from build123d import *

# Parameters (mm, degrees)
SKETCH1_R           = 5
BOSS_EXTRUDE1_DEPTH = 40
SKETCH1_3_R         = 7.5
SKETCH1_3_R_2       = 5
BOSS_EXTRUDE2_DEPTH = 3
SKETCH2_R           = 7.5
BOSS_EXTRUDE3_DEPTH = 7


with BuildPart() as part:
    # Sketch1 → Boss-Extrude1 (new body)
    with BuildSketch(Plane(origin=(0, 0, 0), x_dir=(1, 0, 0), z_dir=(0, 1, 0))):
        with Locations(Location((0, 0, 0), (0, 0, 270))):
            Circle(SKETCH1_R)
    extrude(amount=BOSS_EXTRUDE1_DEPTH)

    # Sketch1_3 → Boss-Extrude2 (add)
    with BuildSketch(Plane(origin=(0, 0, 0), x_dir=(1, 0, 0), z_dir=(0, 1, 0))):
        with Locations(Location((0, 0, 0), (0, 0, 270))):
            Circle(SKETCH1_3_R)
        Polygon((2.886751346, -5), (5.773502692, 0), (2.886751346, 5), (-2.886751346, 5), (-5.773502692, 0), (-2.886751346, -5), align=None, mode=Mode.SUBTRACT)
        with BuildLine():
            ThreePointArc((-4.330127013, 2.500000011), (-2.499999995, 4.330127022), (0, 5))
            Line((0, 5), (-2.886751346, 5))
            Line((-2.886751346, 5), (-4.330127013, 2.500000011))
        make_face()
        with BuildLine():
            ThreePointArc((0, 5), (2.500000021, 4.330127007), (4.330127043, 2.499999958))
            Line((4.330127043, 2.499999958), (2.886751346, 5))
            Line((2.886751346, 5), (0, 5))
        make_face()
        with BuildLine():
            Line((4.330126994, -2.500000043), (5.773502692, 0))
            Line((5.773502692, 0), (4.330127043, 2.499999958))
            ThreePointArc((4.330127043, 2.499999958), (4.829629138, 1.294095202), (5, 0))
            ThreePointArc((5, 0), (4.829629125, -1.294095249), (4.330126994, -2.500000043))
        make_face()
        with BuildLine():
            Line((2.886751346, -5), (4.330126994, -2.500000043))
            ThreePointArc((4.330126994, -2.500000043), (2.499999979, -4.330127031), (0, -5))
            Line((0, -5), (2.886751346, -5))
        make_face()
        with BuildLine():
            Line((-2.886751346, -5), (0, -5))
            ThreePointArc((0, -5), (-2.499999995, -4.330127022), (-4.330127013, -2.500000011))
            Line((-4.330127013, -2.500000011), (-2.886751346, -5))
        make_face()
        with BuildLine():
            ThreePointArc((-4.330127013, -2.500000011), (-5, 0), (-4.330127013, 2.500000011))
            Line((-4.330127013, 2.500000011), (-5.773502692, 0))
            Line((-5.773502692, 0), (-4.330127013, -2.500000011))
        make_face()
        with Locations(Location((0, 0, 0), (0, 0, 270))):
            Circle(SKETCH1_3_R_2)
    extrude(amount=-BOSS_EXTRUDE2_DEPTH)

    # Sketch2 → Boss-Extrude3 (add)
    with BuildSketch(Plane.XZ.offset(3)):
        with Locations(Location((0, 0, 0), (0, 0, 90))):
            Circle(SKETCH2_R)
        Polygon((5.773502692, 0), (2.886751346, 5), (-2.886751346, 5), (-5.773502692, 0), (-2.886751346, -5), (2.886751346, -5), align=None, mode=Mode.SUBTRACT)
    extrude(amount=BOSS_EXTRUDE3_DEPTH)


solid = part.part
Verification items for the finished model (mm, model axes). A direction names the side the tool comes from. Coordinates: 2 decimals unless noted, no trailing zeros. Order: outer loops, then holes, each group sorted by start corner. A loop starts at its lowest first (then second) coordinate and runs counter-clockwise, first axis right, second up. Notation, with made-up numbers: (-11, 18) -> (4, 18) arc R34 cw to (4, 54) -> close; hole circle Ø3 at (83.5, 3). An arc over 180 degrees is marked (long way). Put each result on its own line as item: value. Start each with the question number.
1. Cross-section at B-B, the plane y = 9. Record the boundary of the cut face in (x, z).
2. Access from +Z, -Z, +X, -X, +Y, -Y to the whole of each face (thin tool, end or side, straight path). Record for faces 5 (the cylindrical face through (-0.33, -4.93, -7.493)), 6 (the flat face through (-5, 0, 2)), 7 (the flat face through (-4.35, -6.451, -2.465)).
3. Material ranges on L1, parallel to Y at x = -1.25, z = -2.75; L2, parallel to Y at x = 4, z = -5; L3, parallel to Z at x = -0.75, y = -6.5, recorded low to high. Write a range as [from, to].
4. Mould release check, pull along Z, two halves, no side actions. Record for faces 1 (the flat face through (0, -6, 5)), 2 (the cylindrical face through (-4.88, 19.72, -1.08)), 3 (the flat face through (4.31, -6.451, -2.535)), 4 (the flat face through (5, -10, -2)): released by +Z, released by -Z, zero draft, split by the parting line, or undercut.
5. Go/stop test with flat-tipped pins: pin 1 Ø5 at (x, y) = (-3, 26) entering from +Z; pin 2 Ø4 at (x, z) = (-5, -6) entering from +Y; pin 3 Ø1.7 at (x, y) = (-1.5, -5) entering from -Z. Record where each tip stops, or that it passes through.
6. Cross-section at D-D, the plane y = -2.5. Record the boundary of the cut face in (x, z), then the cut area to 3 significant figures.
7. Cross-section at C-C, the plane z = -6.25. Record the boundary of the cut face in (x, y), then the cut area to 3 significant figures.
8. Cross-section at A-A, the plane x = 0. Record the boundary of the cut face in (y, z), then the cut area to 3 significant figures.
Computed:
1. outline: circle Ø10 at (0, 0)
2. face 5: +Y, -Y
2. face 6: +Y
2. face 7: -Y
3. L1: [-3, 40]
3. L2: [-10, 0]
3. L3: [-7.46, -5], [5, 7.46]
4. face 1: undercut
4. face 2: split by the parting line
4. face 3: undercut
4. face 4: zero draft
5. pin 1: z = 4.97
5. pin 2: y = 0
5. pin 3: z = -7.47
6. outline: circle Ø15 at (0, 0)
6. area: 177 mm2
7. outline: (-4.15, -10) -> (4.15, -10) -> (4.15, 0) -> (-4.15, 0) -> close
7. area: 82.9 mm2
8. outline: (-10, -7.5) -> (0, -7.5) -> (0, -5) -> (40, -5) -> (40, 5) -> (0, 5) -> (0, 7.5) -> (-10, 7.5) -> (-10, 5) -> (-3, 5) -> (-3, -5) -> (-10, -5) -> close
8. area: 480 mm2
